Here's how the part is built. I have some questions about the finished solid (model axes, mm). Face numbers are marked on the shaded views. A direction names the side the tool comes from. Give positions to 0.01 mm unless a question says otherwise; leave off trailing zeros. Loops run counter-clockwise (first coordinate to the right, second up) from the corner with the lowest first, then second, coordinate; pieces in that order, holes last.
Q1. I need wall thicknesses on probe 1 along Z at (x, y) = (-21, 73); probe 2 along X at (y, z) = (53, 11); probe 3 along Y at (x, z) = (-43, 8.5). Which ranges of each line are inside material? Lowest first, please.
Q2. Suppose I cut it at B-B (y = 37). List the corners of the cut face in (x, z) for me, and give its area (3 significant figures).
Q3. Suppose I cut it at D-D (x = -38). List the corners of the cut face in (y, z) for me.
Q4. I'm going to push flat-ended pins straight in: P1, Ø2, axis at y = 85.5, z = -34.5, coming from the +X side; P2, Ø6, axis at y = 61, z = 11.5, coming from the -X side; P3, Ø2.5, axis at x = -10, y = 74.5, coming from the +Z side; P4, Ø10, axis at y = 75.5, z = 14.5, coming from the +X side. Where does each tip first touch, or does it pass through?
Q5. Suppose I cut it at A-A (x = -31). List the corners of the cut face in (y, z) for me.
Q6. For the marked faces 1 and 2, which set-ups out of +Z, -Z, +X, -X, +Y, -Y let a thin tool reach every point of the face, with its end or its side?
Q7. Suppose I cut it at C-C (z = 8.5). List the corners of the cut face in (x, y) for me.
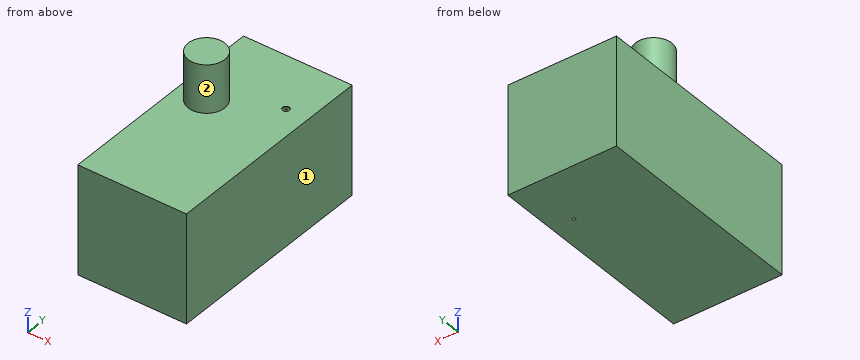
```python
from build123d import *

# Parameters (mm, degrees)
SKETCH1_W                                           = 50
SKETCH1_H                                           = 50
BOSS_EXTRUDE1_DEPTH                                 = 100
SKETCH2_R                                           = 8.427155927
BOSS_EXTRUDE2_DEPTH                                 = 22
CBORE_FOR_00_BINDING_HEAD_MACHINE_SCREW_D           = 1.397
CBORE_FOR_00_BINDING_HEAD_MACHINE_SCREW_CBORE_D     = 3.175
CBORE_FOR_00_BINDING_HEAD_MACHINE_SCREW_CBORE_DEPTH = 0.7112


with BuildPart() as part:
    # Sketch1 → Boss-Extrude1 (new body)
    with BuildSketch(Plane(origin=(0, 0, 0), x_dir=(1, 0, 0), z_dir=(0, 1, 0))):
        with Locations((-25, 25)):
            Rectangle(SKETCH1_W, SKETCH1_H)
    extrude(amount=BOSS_EXTRUDE1_DEPTH)

    # Sketch2 → Boss-Extrude2 (add)
    with BuildSketch(Plane.XY):
        with Locations((-36.936942804, 60.539744496)):
            Circle(SKETCH2_R)
    extrude(amount=BOSS_EXTRUDE2_DEPTH)

    # CBORE for #00 Binding Head Machine Screw1 (through all)
    with Locations(Plane.XY):
        with Locations((-10.367880278, 73.678854219)):
            CounterBoreHole(CBORE_FOR_00_BINDING_HEAD_MACHINE_SCREW_D / 2, CBORE_FOR_00_BINDING_HEAD_MACHINE_SCREW_CBORE_D / 2, CBORE_FOR_00_BINDING_HEAD_MACHINE_SCREW_CBORE_DEPTH)


solid = part.part
```
Solutions:
1. probe 1: z = -50 to 0
1. probe 2: x = -40.7 to -33.17
1. probe 3: y = 54.69 to 66.39
2. outline: (-50, -50) - (0, -50) - (0, 0) - (-50, 0) - close
2. area: 2,500 mm2
3. outline: (0, -50) - (100, -50) - (100, 0) - (68.9, 0) - (68.9, 22) - (52.18, 22) - (52.18, 0) - (0, 0) - close
4. P1: stops at x = 0
4. P2: stops at x = -45.36
4. P3: stops at z = 0
4. P4: passes through
5. outline: (0, -50) - (100, -50) - (100, 0) - (66.52, 0) - (66.52, 22) - (54.56, 22) - (54.56, 0) - (0, 0) - close
6. face 1: +Z, -Z, +X, +Y, -Y
6. face 2: +Z
7. outline: circle Ø16.85 at (-36.94, 60.54)
